from build123d import *

# Parameters (mm, degrees)
F0_R     = 17.5
F0_W     = 10
F0_H     = 30
F0_W_2   = 8
F0_H_2   = 15
F1_DEPTH = 15


# Not quite as in the source:
# - a feature of the source that left no trace in its solid (it failed there, or was rolled back) is left out


with BuildPart() as f1:
    # F0 (on Top) → F1 (new body)
    with BuildSketch(Plane.XY):
        with BuildLine():
            Line((60.2198065221, 40), (-94.7801934779, 40))
            Line((-94.7801934779, 40), (-94.7801934779, 15))
            Line((-94.7801934779, 15), (-94.4899649718, 15))
            Line((-94.4899649718, 15), (-84.4899649718, 15))
            Line((-84.4899649718, 15), (-74.4899649718, 15))
            Line((-74.4899649718, 15), (-66.4899649718, 15))
            Line((-66.4899649718, 15), (-56.4899649718, 15))
            Line((-56.4899649718, 15), (-42.4899649718, 15))
            Line((-42.4899649718, 15), (60.2198065221, 15))
            ThreePointArc((60.2198065221, 15), (127.9115485987, 27.5), (60.2198065221, 40))
        make_face()
        with Locations((92.9115485987, 27.5)):
            Circle(F0_R, mode=Mode.SUBTRACT)
        with Locations((-89.4899649718, 0)):
            Rectangle(F0_W, F0_H)
        with Locations((-70.4899649718, 7.5)):
            Rectangle(F0_W_2, F0_H_2)
        Polygon((-49.4899649718, 0), (-42.4899649718, 15), (-56.4899649718, 15), align=None)
    extrude(amount=F1_DEPTH)


solid = f1.part
CAD build for the part. Positions are in the model's coordinates, mm. A direction names the side the tool comes from. Give positions to 0.01 mm unless a question says otherwise; leave off trailing zeros. Order: outer loops, then holes, each group sorted by start corner. A loop starts at its lowest first (then second) coordinate and runs counter-clockwise, first axis right, second up. Notation, with made-up numbers: (6.5, 18) - (41.5, 18) arc R31 ccw to (41.5, 56) - close; hole circle Ø6 at (26, -3.75). An arc over 180 degrees is marked (long way). Write each question's results on one line, items separated by ' | '.
1. Pin check, flat tips, straight feed: pin 1 (5 mm diameter, centred on x = -78, z = 10, fed in from -Y); pin 2 (7.5 mm diameter, centred on y = 5, z = 7, fed in from -X); pin 3 (1 mm diameter, centred on y = 5.5, z = 4, fed in from +X). Stop position of each tip, or through.
Calculated:
pin 1: stops at y = 15 | pin 2: stops at x = -94.49 | pin 3: stops at x = 120.53
2. Pull direction X, two halves, no side cores. Call faces 1 (the face through (-16, 40, 7)), 2 (the face through (-94.49, 0, 7)), 3 (the face through (-53.039, 7.605, 7.395)): released by +X, released by -X, zero draft, split by the parting line, or undercut.
Calculated:
face 1: zero draft | face 2: released by -X | face 3: undercut
3. Saw through at A-A on y = 27.5. List the corners of the cut face in (x, z).
Calculated:
outline: (-94.78, 0) - (75.41, 0) - (75.41, 15) - (-94.78, 15) - close; (110.41, 0) - (127.91, 0) - (127.91, 15) - (110.41, 15) - close
4. Saw through at B-B on z = 4.75. List the corners of the cut face in (x, y).
Calculated:
outline: (-94.78, 15) - (-94.49, 15) - (-94.49, -15) - (-84.49, -15) - (-84.49, 15) - (-74.49, 15) - (-74.49, 0) - (-66.49, 0) - (-66.49, 15) - (-56.49, 15) - (-49.49, 0) - (-42.49, 15) - (60.22, 15) arc R35 ccw (long way) to (60.22, 40) - (-94.78, 40) - close; hole circle Ø35 at (92.91, 27.5)
5. Saw through at C-C on x = 108.5. List the corners of the cut face in (y, z), and give its area (3 significant figures).
Calculated:
outline: (-3.84, 0) - (19.55, 0) - (19.55, 15) - (-3.84, 15) - close; (35.45, 0) - (58.84, 0) - (58.84, 15) - (35.45, 15) - close | area: 702 mm2
6. Saw through at D-D on x = 32.5. List the corners of the cut face in (y, z), and give its area (3 significant figures).
Calculated:
outline: (15, 0) - (40, 0) - (40, 15) - (15, 15) - close | area: 375 mm2
7. Probe L1, parallel to Y at x = -85, z = 7.25; L2, parallel to Y at x = -40, z = 8.75; L3, parallel to X at y = 32, z = 5.5. List the from-to ranges inside material, lowest first. Write a range as from..to.
Calculated:
L1: y = -15..40 | L2: y = 15..40 | L3: x = -94.78..76, 109.82..127.62
8. 3-axis set-ups, long thin cutter, end or side, ignore diameter. For faces 4 (the face through (-94.78, 28, 7)), 5 (the face through (-62, 15, 7)): which of +Z, -Z, +X, -X, +Y, -Y reach the whole face in a straight line?
Calculated:
face 4: +Z, -Z, -X, +Y, -Y | face 5: +Z, -Z, -Y
